from build123d import *

# Parameters (mm, degrees)
SKETCH1_W           = 6
SKETCH1_H           = 8
BOSS_EXTRUDE1_DEPTH = 5.1
BOSS_EXTRUDE2_DEPTH = 5.1
SKETCH3_W           = 4
SKETCH3_H           = 0.55
BOSS_EXTRUDE3_DEPTH = 3.5


with BuildPart() as part:
    # Sketch1 → Boss-Extrude1 (new body)
    with BuildSketch(Plane(origin=(0, 0, 0), x_dir=(1, 0, 0), z_dir=(0, 1, 0))):
        Rectangle(SKETCH1_W, SKETCH1_H)
    extrude(amount=BOSS_EXTRUDE1_DEPTH)

    # Sketch2 → Boss-Extrude2 (add)
    with BuildSketch(Plane.XZ):
        Polygon((3, -6), (-3, -6), (-3, -5.2), (-1.8, -4), (1.8, -4), (3, -5.2), align=None)
    extrude(amount=-BOSS_EXTRUDE2_DEPTH)

    # Sketch3 → Boss-Extrude3 (add)
    with BuildSketch(Plane.XZ):
        with Locations((0, 2.625)):
            Rectangle(SKETCH3_W, SKETCH3_H)
    extrude(amount=BOSS_EXTRUDE3_DEPTH)


solid = part.part
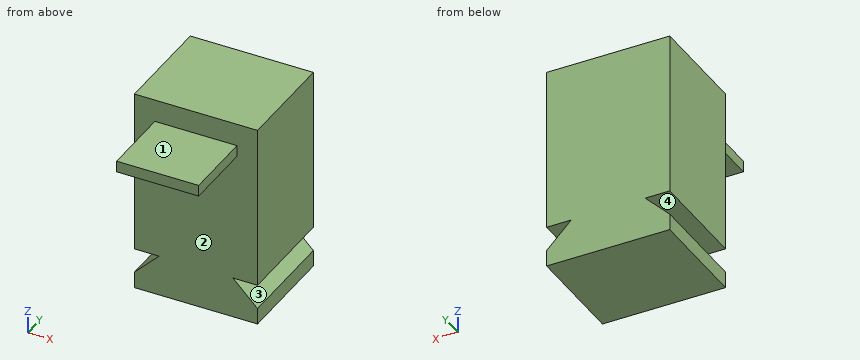
Verification items for the finished model (mm, model axes). Face numbers are marked on the shaded views. Give positions to 0.01 mm unless a question says otherwise; leave off trailing zeros. Write each loop counter-clockwise with the first axis right and the second up, starting at its lowest first coordinate (ties: lowest second). Pieces come first, ordered by that corner, then holes. Notation, with made-up numbers: (36, 61.25) - (86, 61.25) arc R30 ccw to (86, 88.25) - close; hole circle Ø1 at (33.25, 1). An arc over 180 degrees is marked (long way). Answer as CSV lines item,"result". Start each with the question number.
1. Thickness scan on line 1 (Y direction, x = 1.7, z = -5.5); line 2 (Z direction, x = 2.5, y = 2.5); line 3 (Z direction, x = -0.35, y = -1). Record the ranges inside material, lowest first.
2. Sectioned sample at B-B (y = 0.75). Record the boundary of the cut face in (x, z), then the cut area to 3 significant figures.
3. Depth check by flat-ended pin: pin 1 (0.6 mm diameter, centred on y = -1, z = 2.5, fed in from -X); pin 2 (5 mm diameter, centred on y = -2, z = 1.5, fed in from +X). Enter the tip coordinate at first touch or a pass-through.
4. Sectioned sample at D-D (x = -0.6). Record the boundary of the cut face in (y, z).
5. Sectioned sample at C-C (z = 2.75). Record the boundary of the cut face in (x, y).
6. Draft check along Z on the marked faces 1, 2, 3 and 4. Enter one of: pulls with the +Z half, pulls with the -Z half, needs draft (parallel to the pull), parting line crosses it, or undercut.
7. Sectioned sample at A-A (x = 2.65). Record the boundary of the cut face in (y, z), then the cut area to 3 significant figures.
Derived:
1,line 1,"0 to 5.1"
1,line 2,"-6 to -4.7, -4 to 4"
1,line 3,"2.35 to 2.9"
2,outline,"(-3, -6) - (3, -6) - (3, -5.2) - (1.8, -4) - (3, -4) - (3, 4) - (-3, 4) - (-3, -4) - (-1.8, -4) - (-3, -5.2) - close"
2,area,"58.6 mm²"
3,pin 1,"x = -2"
3,pin 2,"x = 3"
4,outline,"(-3.5, 2.35) - (0, 2.35) - (0, -6) - (5.1, -6) - (5.1, 4) - (0, 4) - (0, 2.9) - (-3.5, 2.9) - close"
5,outline,"(-3, 0) - (-2, 0) - (-2, -3.5) - (2, -3.5) - (2, 0) - (3, 0) - (3, 5.1) - (-3, 5.1) - close"
6,face 1,"pulls with the +Z half"
6,face 2,"needs draft"
6,face 3,"undercut"
6,face 4,"undercut"
7,outline,"(0, -6) - (5.1, -6) - (5.1, -4.85) - (0, -4.85) - close; (0, -4) - (5.1, -4) - (5.1, 4) - (0, 4) - close"
7,area,"46.7 mm²"
